Model file for the job. Use its own axes, mm. A direction names the side the tool comes from. Round coordinates to 2 decimals unless told otherwise and drop trailing zeros. Order: outer loops, then holes, each group sorted by start corner. A loop starts at its lowest first (then second) coordinate and runs counter-clockwise, first axis right, second up. Notation, with made-up numbers: (56, -19) - (83, -19) arc R11 ccw to (83, -1) - close; hole circle Ø1 at (-10, 87). An arc over 180 degrees is marked (long way). Write item = value, one per line. Start each with the question number.
from build123d import *

# Parameters (mm, degrees)
F1_DEPTH = 38.1
F2_R     = 1.27
F3_R     = 2.54
F4_DEPTH = 2.794
F5_R     = 2.54
F6_DEPTH = 2.794


with BuildPart() as f1:
    # F0 (on Right) → F1 (new body)
    with BuildSketch(Plane.YZ):
        with BuildLine():
            Line((-2.794, 0), (0, 0))
            Line((0, 0), (0, 36.576))
            ThreePointArc((0, 36.576), (-1.562292, 40.347708), (-5.334, 41.91))
            Line((-5.334, 41.91), (-37.084, 41.91))
            Line((-37.084, 41.91), (-37.084, 39.116))
            Line((-37.084, 39.116), (-5.334, 39.116))
            ThreePointArc((-5.334, 39.116), (-3.537949, 38.372051), (-2.794, 36.576))
            Line((-2.794, 36.576), (-2.794, 0))
        make_face()
    extrude(amount=F1_DEPTH)

    # F2
    f2_edges = [f1.edges().sort_by_distance(p)[0] for p in [
        (0, -37.084, 40.513),
        (38.1, -37.084, 40.513),
        (38.1, -1.397, 0),
        (0, -1.397, 0),
    ]]
    fillet(f2_edges, radius=F2_R)

    # F3 (on face) → F4 (cut, through all)
    with BuildSketch(Plane.XY.offset(41.91)):
        with Locations((19.05, -25.019)):
            Circle(F3_R)
    extrude(amount=-F4_DEPTH, mode=Mode.SUBTRACT)

    # F5 (on face) → F6 (cut, through all)
    with BuildSketch(Plane.XZ.offset(2.794)):
        with Locations((28.575, 27.051)):
            Circle(F5_R)
        with Locations((9.525, 9.525)):
            Circle(F5_R)
    extrude(amount=-F6_DEPTH, mode=Mode.SUBTRACT)


solid = f1.part
Item 1: Probe L1, parallel to Z at x = 25, y = -26; L2, parallel to Y at x = 14.5, z = 17; L3, parallel to Y at x = 19.05, z = 39.85. List the from-to ranges inside material, lowest first.
Item 2: Saw through at D-D, the plane y = -20. Give the cut face in (x, z).
Item 3: Saw through at C-C, the plane x = 32. Give the cut face in (y, z).
Item 4: Drop flat-ended pins along their axis: pin 1 (4 mm diameter, centred on x = 33.5, y = -30, fed in from -Z); pin 2 (1.5 mm diameter, centred on x = 11, z = 5.5, fed in from -Y); pin 3 (10 mm diameter, centred on x = 12.5, z = 34.5, fed in from -Y). Give the stop position or say it passes through.
Item 5: Saw through at B-B, the plane z = 28.5. Give the cut face in (x, y).
Item 6: Mould opens along X. For faces 3 (the face through (37.718, -1.377, 0.362)), 4 (the face through (7.51, -1.42, 7.98)), 5 (the face through (19, -21, 39.116)) say: +X half, -X half, draft (parallel to the pull), parting line (faces both ways), or undercut.
Item 7: Saw through at A-A, the plane x = 19.05. Give the cut face in (y, z).
Item 8: Which spindle directions (+Z, -Z, +X, -X, +Y, -Y) get a long thin tool onto all of the face, cutting with end or side? Do faces 1 (the face through (19, -2.794, 19)), 2 (the face through (37.72, -36.72, 40.49)). Say none if no direction does.
Check sheet entries:
q1.L1 = 39.12 to 41.91
q1.L2 = -2.79 to 0
q1.L3 = -37.08 to -27.56, -22.48 to -1.12
q2.outline = (0, 39.12) - (38.1, 39.12) - (38.1, 41.91) - (0, 41.91) - close
q3.outline = (-37.08, 39.12) - (-5.33, 39.12) arc R2.54 cw to (-2.79, 36.58) - (-2.79, 0) - (0, 0) - (0, 36.58) arc R5.33 ccw to (-5.33, 41.91) - (-37.08, 41.91) - close
q4.pin_1 = 39.12
q4.pin_2 = -2.79
q4.pin_3 = -37.08
q5.outline = (0, -2.79) - (26.49, -2.79) - (26.49, 0) - (0, 0) - close; (30.66, -2.79) - (38.1, -2.79) - (38.1, 0) - (30.66, 0) - close
q6.face_3 = +X half
q6.face_4 = undercut
q6.face_5 = draft
q7.outline = (-37.08, 39.12) - (-27.56, 39.12) - (-27.56, 41.91) - (-37.08, 41.91) - close; (-22.48, 39.12) - (-5.33, 39.12) arc R2.54 cw to (-2.79, 36.58) - (-2.79, 0) - (0, 0) - (0, 36.58) arc R5.33 ccw to (-5.33, 41.91) - (-22.48, 41.91) - close
q8.face_1 = -Z, +X, -X, -Y
q8.face_2 = +Z, -Z, +X, -Y
